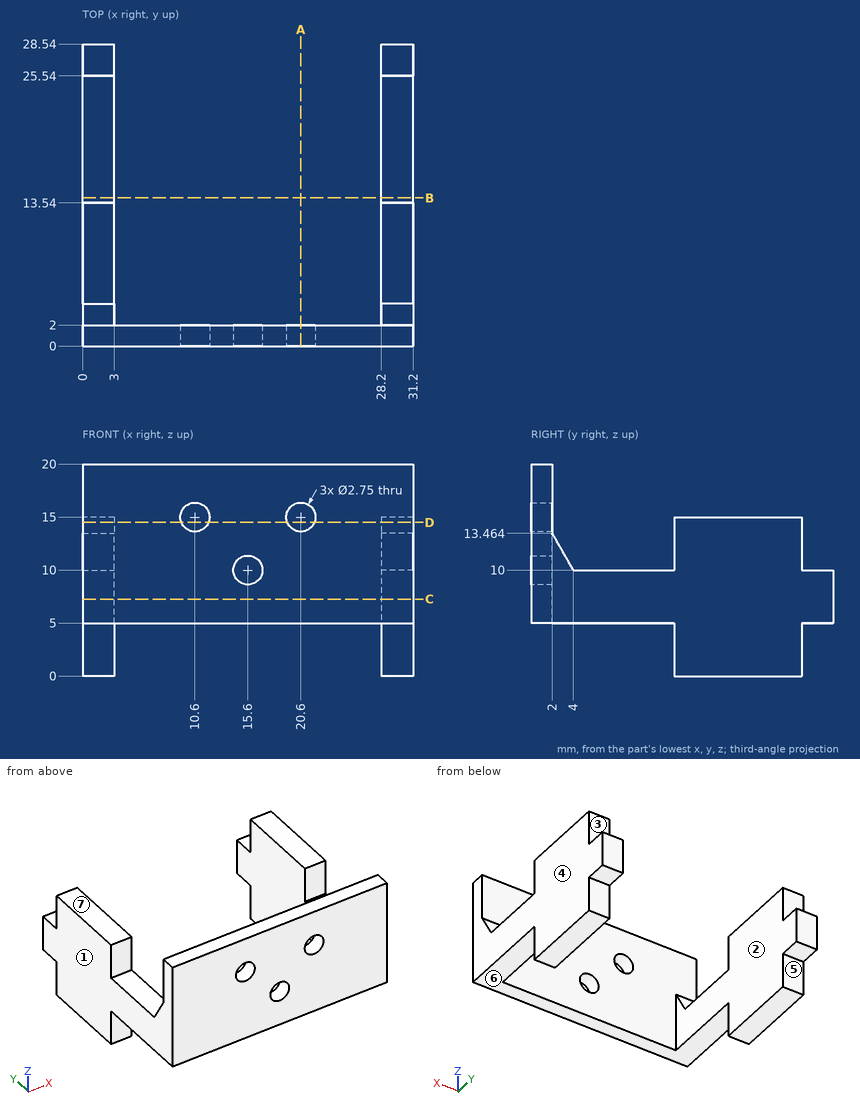
Check sheet for the drawn part. Datum: minimum x, y, z corner. Units: mm. A direction names the side the tool comes from. Round coordinates to 2 decimals unless told otherwise and drop trailing zeros. Order: outer loops, then holes, each group sorted by start corner. A loop starts at its lowest first (then second) coordinate and runs counter-clockwise, first axis right, second up. Notation, with made-up numbers: (70.5, -3.75) -> (114.5, -3.75) arc R25 ccw to (114.5, 34.25) -> close; hole circle Ø6 at (-6, 12.25). An arc over 180 degrees is marked (long way). Put each result on its own line as item: value. Start each with the question number.
(1) Tool access check on the marked faces 5, 6 and 7. Record the directions out of +Z, -Z, +X, -X, +Y, -Y that give a thin tool (end or side, any length) a straight path to the whole face; none if there is none.
(2) Section check D-D (z = 14.5). Enter the section's corners in (x, y), then the cut area to 3 significant figures.
(3) Depth check by flat-ended pin: pin 1 Ø7.5 at (x, z) = (11, 9) entering from +Y; pin 2 Ø0.9 at (x, z) = (30, 2.5) entering from -Y; pin 3 Ø12 at (y, z) = (7, 2) entering from +X; pin 4 Ø1.5 at (x, y) = (29, 19) entering from +Z. Enter the tip coordinate at first touch or a pass-through.
(4) Section check C-C (z = 7.25). Enter the section's corners in (x, y).
(5) Section check A-A (x = 20.6). Enter the section's corners in (y, z) (3 decimals).
(6) Draft check along X on the marked faces 1, 2, 3 and 4. Enter one of: +X half, -X half, draft (parallel to the pull), parting line (faces both ways), or undercut.
(7) Material ranges on line 1 along X through (y, z) = (1.4, 15) (3 decimals); line 2 along X through (y, z) = (23, 9.5); line 3 along Y through (x, z) = (10.5, 5.25), recorded low to high.
(8) Section check B-B (y = 14). Enter the section's corners in (x, z), then the cut area to 3 significant figures.
Completed:
1. face 5: -Z, +X, -X, +Y
1. face 6: -Z, +X, -X, -Y
1. face 7: +Z, +X, -X, +Y
2. outline: (0, 0) -> (9.32, 0) -> (9.32, 2) -> (0, 2) -> close; (0, 13.54) -> (3, 13.54) -> (3, 25.54) -> (0, 25.54) -> close; (11.88, 0) -> (19.32, 0) -> (19.32, 2) -> (11.88, 2) -> close; (21.88, 0) -> (31.2, 0) -> (31.2, 2) -> (21.88, 2) -> close; (28.2, 13.54) -> (31.2, 13.54) -> (31.2, 25.54) -> (28.2, 25.54) -> close
2. area: 124 mm2
3. pin 1: stops at y = 2
3. pin 2: stops at y = 13.54
3. pin 3: stops at x = 31.2
3. pin 4: stops at z = 15
4. outline: (0, 0) -> (31.2, 0) -> (31.2, 28.54) -> (28.2, 28.54) -> (28.2, 2) -> (3, 2) -> (3, 28.54) -> (0, 28.54) -> close
5. outline: (0, 5) -> (2, 5) -> (2, 13.625) -> (0, 13.625) -> close; (0, 16.375) -> (2, 16.375) -> (2, 20) -> (0, 20) -> close
6. face 1: -X half
6. face 2: undercut
6. face 3: draft
6. face 4: +X half
7. line 1: x = 0 to 9.225, 11.975 to 19.225, 21.975 to 31.2
7. line 2: x = 0 to 3, 28.2 to 31.2
7. line 3: y = 0 to 2
8. outline: (0, 0) -> (3, 0) -> (3, 15) -> (0, 15) -> close; (28.2, 0) -> (31.2, 0) -> (31.2, 15) -> (28.2, 15) -> close
8. area: 90.0 mm2
